Read the model definition and answer for the solid it produces. Units are mm, in the model's axes. Give positions to 0.01 mm unless a question says otherwise; leave off trailing zeros. Loops run counter-clockwise (first coordinate to the right, second up) from the corner with the lowest first, then second, coordinate; pieces in that order, holes last. Notation, with made-up numbers: (34, 32) -> (75, 32) arc R21 cw to (75, 56) -> close; hole circle Ø5 at (57.25, 57.5). An arc over 180 degrees is marked (long way). Write each question's results on one line, items separated by ' | '. Start each with the question number.
Item 1: Section A-A on z = 216 is taken. Write down the section's boundary in (x, y) (3 decimals).
Item 2: Find the intervals of material crossed by line 1 (Y direction, x = 0, z = 19.5) (3 decimals); line 2 (X direction, y = -11.5, z = 46) (3 decimals); line 3 (Y direction, x = 4, z = 134), in increasing order.
Item 3: Section C-C on y = -17.5 is taken. Write down the section's boundary in (x, z) (3 decimals).
Item 4: Section D-D on z = 34.5 is taken. Write down the section's boundary in (x, y) (3 decimals), and give its area (3 significant figures).
Item 5: Section B-B on x = 0 is taken. State how many separate pieces and enclosed holes the cut face has, and give its area (3 significant figures).
Item 6: Each of these flat-tipped pins is pushed along its axis until it touches: P1, Ø1.8, axis at x = 3.5, z = 297, coming from the +Y side; P2, Ø2, axis at x = 0.5, y = -22.5, coming from the +Z side (3 decimals); P3, Ø5.5, axis at x = 2, y = -4, coming from the +Z side; P4, Ø17, axis at y = -21, z = 274.5, coming from the -X side (3 decimals). Where does it stop, or does it pass through?
```python
from build123d import *

# Parameters (mm, degrees)
SKETCH1_R           = 3.175
BOSS_EXTRUDE1_DEPTH = 406.4
SKETCH2_W           = 25.4
SKETCH2_H           = 12.7
CUT_EXTRUDE1_DEPTH  = 11.922
LPATTERN1_COUNT     = 8
LPATTERN1_PITCH     = 50.8


with BuildPart() as part:
    # Sketch1 → Boss-Extrude1 (new body)
    with BuildSketch(Plane.XY):
        with BuildLine():
            Line((5.461, 0), (5.461, -38.1))
            Line((5.461, -38.1), (3.175, -38.1))
            Line((3.175, -38.1), (3.175, -4.443185344))
            ThreePointArc((3.175, -4.443185344), (-4.855985791, 2.498384078), (5.461, 0))
        make_face()
        Circle(SKETCH1_R, mode=Mode.SUBTRACT)
    extrude(amount=BOSS_EXTRUDE1_DEPTH)

    # Sketch2 → Cut-Extrude1 (cut, through all)
    with BuildSketch(Plane(origin=(5.461, 0, 0), x_dir=(0, 0, -1), z_dir=(1, 0, 0))):
        with Locations((-393.7, -0.889)):
            Rectangle(SKETCH2_W, SKETCH2_H)
    cut_extrude1 = extrude(amount=-CUT_EXTRUDE1_DEPTH, mode=Mode.SUBTRACT)

    # LPattern1: Cut-Extrude1 ×8
    with Locations(*[(0, 0, -i * LPATTERN1_PITCH) for i in range(1, LPATTERN1_COUNT)]):
        add(cut_extrude1, mode=Mode.SUBTRACT)


solid = part.part
```
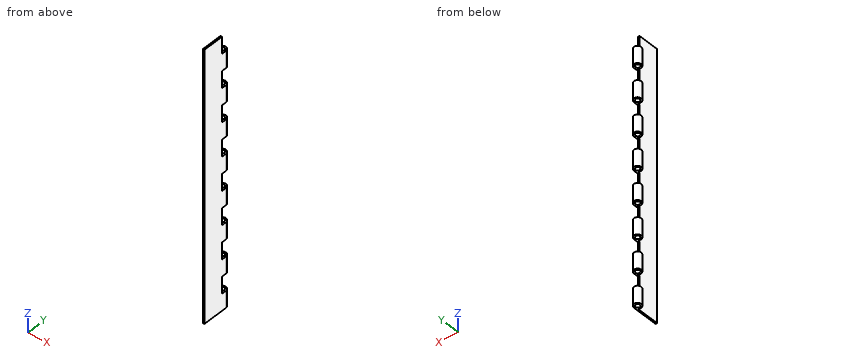
Findings:
1) outline: (3.175, -38.1) -> (5.461, -38.1) -> (5.461, 0) arc R5.461 ccw (long way) to (3.175, -4.443) -> close; hole circle Ø6.35 at (0, 0)
2) line 1: -5.461 to -3.175, 3.175 to 5.461 | line 2: 3.175 to 5.461 | line 3: -38.1 to -7.24
3) outline: (3.175, 0) -> (5.461, 0) -> (5.461, 406.4) -> (3.175, 406.4) -> close
4) outline: (3.175, -38.1) -> (5.461, -38.1) -> (5.461, -7.239) -> (3.175, -7.239) -> close | area: 70.5 mm2
5) separate pieces: 16 | enclosed holes: 0 | area: 929 mm2
6) P1: y = -7.24 | P2: through | P3: z = 381 | P4: x = 3.175
